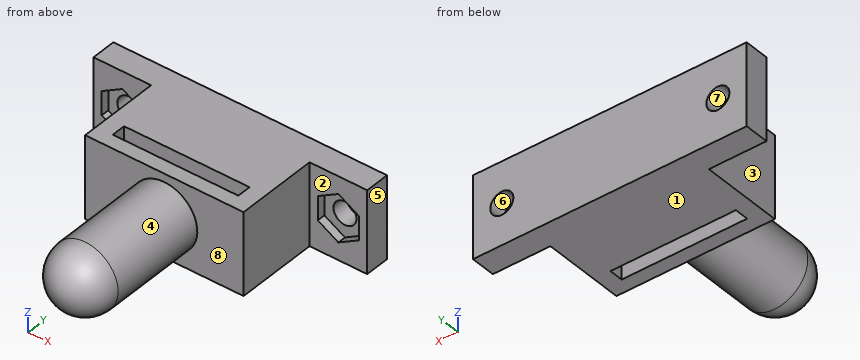
from build123d import *

# Parameters (mm, degrees)
SKETCH1_W             = 7
SKETCH1_H             = 10
BOSS_EXTRUDE1_DEPTH   = 3
BOSS_EXTRUDE1_2_DEPTH = 3
SKETCH1_4_W           = 19.24
SKETCH1_4_H           = 10
BOSS_EXTRUDE2_DEPTH   = 13
SKETCH2_W             = 15.24
SKETCH2_H             = 1.7
CUT_EXTRUDE1_DEPTH    = 14
SKETCH3_R             = 4
BOSS_EXTRUDE3_DEPTH   = 16
FILLET1_R             = 4
CUT_EXTRUDE2_REACH    = 35.797
SKETCH4_R             = 1.4
CUT_EXTRUDE3_REACH    = 37.797
CUT_EXTRUDE3_START    = -2
SKETCH4_3_R           = 1.4


with BuildPart() as part:
    # Sketch1 → Boss-Extrude1 (new body)
    with BuildSketch(Plane(origin=(0, 0, 0), x_dir=(1, 0, 0), z_dir=(0, 1, 0))):
        with Locations((-13.12, 0)):
            Rectangle(SKETCH1_W, SKETCH1_H)
    extrude(amount=-BOSS_EXTRUDE1_DEPTH)



with BuildPart() as body_2:
    # Sketch1 → Boss-Extrude1 2 (new body)
    with BuildSketch(Plane(origin=(0, 0, 0), x_dir=(1, 0, 0), z_dir=(0, 1, 0))):
        with Locations((13.12, 0)):
            Rectangle(SKETCH1_W, SKETCH1_H)
    extrude(amount=-BOSS_EXTRUDE1_2_DEPTH)


with BuildPart() as part_1:
    add(part.part)

    add(body_2.part)  # Boss-Extrude2 merges body 2
    # Sketch1_4 → Boss-Extrude2 (add)
    with BuildSketch(Plane(origin=(0, 0, 0), x_dir=(1, 0, 0), z_dir=(0, 1, 0))):
        Rectangle(SKETCH1_4_W, SKETCH1_4_H)
    extrude(amount=-BOSS_EXTRUDE2_DEPTH)

    # Sketch2 → Cut-Extrude1 (cut)
    with BuildSketch(Plane.XY.offset(5)):
        with Locations((0, -10.45)):
            Rectangle(SKETCH2_W, SKETCH2_H)
    extrude(amount=-CUT_EXTRUDE1_DEPTH, mode=Mode.SUBTRACT)

    # Sketch3 → Boss-Extrude3 (add)
    with BuildSketch(Plane.XZ.offset(13)):
        with Locations(Location((0, 0, 0), (0, 0, 270))):
            Circle(SKETCH3_R)
    extrude(amount=BOSS_EXTRUDE3_DEPTH)

    # Fillet1
    fillet1_edges = [part_1.edges().sort_by_distance(p)[0] for p in [
        (0, -29, 4),
    ]]
    fillet(fillet1_edges, radius=FILLET1_R)

    # Sketch4 → Cut-Extrude2 (cut, up to next)
    with BuildSketch(Plane(origin=(0, 0, 0), x_dir=(1, 0, 0), z_dir=(0, 1, 0)), mode=Mode.PRIVATE) as cut_extrude2_sk1:
        with Locations(Location((-13.12, 0, 0), (0, 0, 270))):
            Circle(SKETCH4_R)
    cut_extrude2_tool1 = extrude(cut_extrude2_sk1.sketch, amount=-CUT_EXTRUDE2_REACH, mode=Mode.PRIVATE) & part_1.part
    # Sketch4 → Cut-Extrude2 (cut, up to next)
    with BuildSketch(Plane(origin=(0, 0, 0), x_dir=(1, 0, 0), z_dir=(0, 1, 0)), mode=Mode.PRIVATE) as cut_extrude2_sk2:
        with Locations(Location((13.12, 0, 0), (0, 0, 270))):
            Circle(SKETCH4_R)
    cut_extrude2_tool2 = extrude(cut_extrude2_sk2.sketch, amount=-CUT_EXTRUDE2_REACH, mode=Mode.PRIVATE) & part_1.part
    add(cut_extrude2_tool1.solids().sort_by_distance((-13.12, 0, 0))[0], mode=Mode.SUBTRACT)
    add(cut_extrude2_tool2.solids().sort_by_distance((13.12, 0, 0))[0], mode=Mode.SUBTRACT)

    # Sketch4_3 → Cut-Extrude3 (cut, up to next)
    with BuildSketch(Plane(origin=(0, 0, 0), x_dir=(1, 0, 0), z_dir=(0, 1, 0)).offset(CUT_EXTRUDE3_START), mode=Mode.PRIVATE) as cut_extrude3_sk1:
        Polygon((-15.62, 1.443375673), (-15.62, -1.443375673), (-13.12, -2.886751346), (-10.62, -1.443375673), (-10.62, 1.443375673), (-13.12, 2.886751346), align=None)
        with Locations(Location((-13.12, 0, 0), (0, 0, 270))):
            Circle(SKETCH4_3_R, mode=Mode.SUBTRACT)
    cut_extrude3_tool1 = extrude(cut_extrude3_sk1.sketch, amount=-CUT_EXTRUDE3_REACH, mode=Mode.PRIVATE) & part_1.part
    # Sketch4_3 → Cut-Extrude3 (cut, up to next)
    with BuildSketch(Plane(origin=(0, 0, 0), x_dir=(1, 0, 0), z_dir=(0, 1, 0)).offset(CUT_EXTRUDE3_START), mode=Mode.PRIVATE) as cut_extrude3_sk2:
        Polygon((10.62, 1.443375673), (10.62, -1.443375673), (13.12, -2.886751346), (15.62, -1.443375673), (15.62, 1.443375673), (13.12, 2.886751346), align=None)
        with Locations(Location((13.12, 0, 0), (0, 0, 270))):
            Circle(SKETCH4_3_R, mode=Mode.SUBTRACT)
    cut_extrude3_tool2 = extrude(cut_extrude3_sk2.sketch, amount=-CUT_EXTRUDE3_REACH, mode=Mode.PRIVATE) & part_1.part
    add(cut_extrude3_tool1.solids().sort_by_distance((-15.543624, -2, 0))[0], mode=Mode.SUBTRACT)
    add(cut_extrude3_tool2.solids().sort_by_distance((10.696376, -2, 0))[0], mode=Mode.SUBTRACT)


solid = part_1.part
Design review of the part built by this model. Coordinates are the model's own, in mm. Face numbers are marked on the shaded views. A direction names the side the tool comes from. Round coordinates to 2 decimals unless told otherwise and drop trailing zeros. Write each loop counter-clockwise with the first axis right and the second up, starting at its lowest first coordinate (ties: lowest second). Pieces come first, ordered by that corner, then holes. Notation, with made-up numbers: (67.5, -10.5) -> (89.5, -10.5) arc R11 cw to (89.5, -2.5) -> close; hole circle Ø1 at (48.5, -12.5). An arc over 180 degrees is marked (long way). One line per item, written item: value. Start each with the question number.
Q1. Add section D-D (z = 3.25). Give the boundary of the cut face in (x, y), then the cut area to 3 significant figures.
Q2. Add section C-C (y = -2.5). Give the boundary of the cut face in (x, z), then the cut area to 3 significant figures.
Q3. The part is to be moulded in two halves that separate along X. For the marked faces 5, 6, 7 and 8, say which applies: pulls with the +X half, pulls with the -X half, needs draft (parallel to the pull), parting line crosses it, or undercut.
Q4. Tool access review of the marked faces 1, 2, 3 and 4: name each direction out of +Z, -Z, +X, -X, +Y, -Y from which nothing blocks a thin tool from reaching the whole face with its end or side.
Q5. Add section A-A (z = 0). State how many separate pieces and enclosed holes the cut face has, then the cut area to 3 significant figures.
Q6. Insertion check: P1, Ø6, axis at y = -19, z = 2, coming from the -X side; P2, Ø3.5, axis at x = 13.12, z = 0, coming from the -Y side; P3, Ø3, axis at y = -9, z = 1, coming from the -X side. Each pin has a flat end and moves straight along its axis. Give the tip position at first contact, or say it passes through.
Q7. To check wall thickness, follow probe 1 along X at (y, z) = (-0.35, 0); probe 2 along Y at (x, z) = (4, -4.25); probe 3 along X at (y, z) = (-11, 1.5). State the ranges of each line that lie inside material, in increasing order.
Q8. Add section B-B (x = 0). Give the boundary of the cut face in (y, z).
Response:
1. outline: (-16.62, -3) -> (-9.62, -3) -> (-9.62, -13) -> (-2.33, -13) -> (-2.33, -25) arc R2.33 ccw to (2.33, -25) -> (2.33, -13) -> (9.62, -13) -> (9.62, -3) -> (16.62, -3) -> (16.62, 0) -> (-16.62, 0) -> close; hole (-7.62, -11.3) -> (7.62, -11.3) -> (7.62, -9.6) -> (-7.62, -9.6) -> close
1. area: 331 mm^2
2. outline: (-16.62, -5) -> (16.62, -5) -> (16.62, 5) -> (-16.62, 5) -> close; hole (-15.62, -1.44) -> (-13.12, -2.89) -> (-10.62, -1.44) -> (-10.62, 1.44) -> (-13.12, 2.89) -> (-15.62, 1.44) -> close; hole (10.62, -1.44) -> (13.12, -2.89) -> (15.62, -1.44) -> (15.62, 1.44) -> (13.12, 2.89) -> (10.62, 1.44) -> close
2. area: 289 mm^2
3. face 5: pulls with the +X half
3. face 6: undercut
3. face 7: undercut
3. face 8: needs draft
4. face 1: -Z, +X, -X, +Y, -Y
4. face 2: +Z, -Z, +X, -Y
4. face 3: +Z, -Z, -X, -Y
4. face 4: -Y
5. separate pieces: 3
5. enclosed holes: 1
5. area: 366 mm^2
6. P1: stops at x = -4
6. P2: stops at y = -2
6. P3: stops at x = -9.62
7. probe 1: x = -16.62 to -14.52, -11.72 to 11.72, 14.52 to 16.62
7. probe 2: y = -13 to -11.3, -9.6 to 0
7. probe 3: x = -9.62 to -7.62, 7.62 to 9.62
8. outline: (-25, -4) -> (-13, -4) -> (-13, -5) -> (-11.3, -5) -> (-11.3, 5) -> (-13, 5) -> (-13, 4) -> (-25, 4) arc R4 ccw to start; (-9.6, -5) -> (0, -5) -> (0, 5) -> (-9.6, 5) -> close
